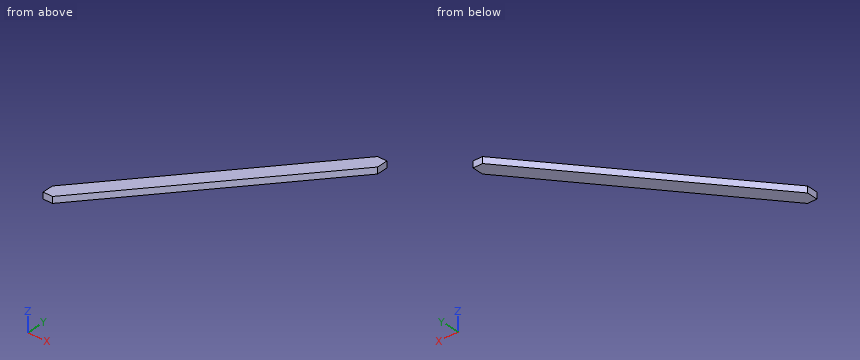
Autodesk Inventor part; units mm, degrees
ref_plane "YZ Plane" through (0, 0, 0) normal (1, 0, 0) x (0, 1, 0)
ref_plane "XZ Plane" through (0, 0, 0) normal (0, 1, 0) x (-1, 0, 0)
ref_plane "XY Plane" through (0, 0, 0) normal (0, 0, 1) x (1, 0, 0)
sketch "Sketch1" plane through (0, 0, 0) normal (0, 0, 1) x (1, 0, 0)
  line L0 (-520.7, -609.6) -> (520.7, -609.6)
  line L1 (520.7, -609.6) -> (520.7, 609.6)
  line L2 (520.7, 609.6) -> (-520.7, 609.6)
  line L3 (-520.7, 609.6) -> (-520.7, -609.6)
  line L4 (-520.7, -609.6) -> (520.7, 609.6) construction
  line L5 (520.7, -609.6) -> (-520.7, 609.6) construction
  line L6 (28.8696, -33.7986) -> (-28.8696, 33.7986)
  line L7 (-520.7, -542.0028) -> (462.9607, 609.6)
  line L8 (-462.9607, -609.6) -> (520.7, 542.0028)
  point P0 (0, 0)
  dimension "d0" = 1219.2
  dimension "d1" = 1041.4
  dimension "d3" = 88.9
extrude "Extrusion1" add sketch "Sketch1" along normal blind 38.1 contours L3 L7 L6 L8 L0 | L6 L7 L2 L1 L8
properties part number "S_2x4x63.127"
Part model, mm, in its own coordinate system. Give positions to 0.01 mm unless a question says otherwise; leave off trailing zeros. Loops run counter-clockwise (first coordinate to the right, second up) from the corner with the lowest first, then second, coordinate; pieces in that order, holes last. Notation, with made-up numbers: M 55,70 L 83,70 A13 ccw 83,95 Z; hole C 58,44.25 d10. An arc over 180 degrees is marked long. Put each result on its own line as item: value. Start each with the question number.
1) Saw through at C-C (x = -355). List the corners of the cut face in (y, z).
2) Saw through at B-B (y = 353). List the corners of the cut face in (x, z).
3) Saw through at A-A (z = 32). List the corners of the cut face in (x, y), then the cut area to 3 significant figures.
4) Flat gauge pins, fed straight in: pin 1 (10 mm diameter, centred on y = 112, z = 10, fed in from +X); pin 2 (8 mm diameter, centred on x = -69.5, z = 18.5, fed in from +Y); pin 3 (1 mm diameter, centred on y = 445, z = 15, fed in from +X). Where does each tip first touch, or does it go through?
5) Probe probe 1 along X at (y, z) = (-462.5, 22); probe 2 along Y at (x, z) = (-411, 4); probe 3 along X at (y, z) = (-233, 5.5). List the from-to ranges inside material, lowest first.
Numbers:
1. outline: M -483.21,0 L -348.01,0 L -348.01,38.1 L -483.21,38.1 Z
2. outline: M 243.78,0 L 359.26,0 L 359.26,38.1 L 243.78,38.1 Z
3. outline: M -520.7,-609.6 L -462.96,-609.6 L 520.7,542 L 520.7,609.6 L 462.96,609.6 L -520.7,-542 Z
3. area: 137,000 mm^2
4. pin 1: x = 157.68
4. pin 2: y = -9.09
4. pin 3: x = 438.27
5. probe 1: -452.79 to -337.31
5. probe 2: -548.77 to -413.57
5. probe 3: -256.76 to -141.28
